Here's the drawing with two shaded views (mm, measured from the low corner). I have some questions. Coordinates: 2 decimals unless noted, no trailing zeros. Write each loop counter-clockwise with the first axis right and the second up, starting at its lowest first coordinate (ties: lowest second). Pieces come first, ordered by that corner, then holes. Notation, with made-up numbers: (-31.75, 76) -> (2.25, 76) arc R33 cw to (2.25, 112) -> close; hole circle Ø7 at (68.25, 30). An arc over 180 degrees is marked (long way). Use one line per item in the form item = value.
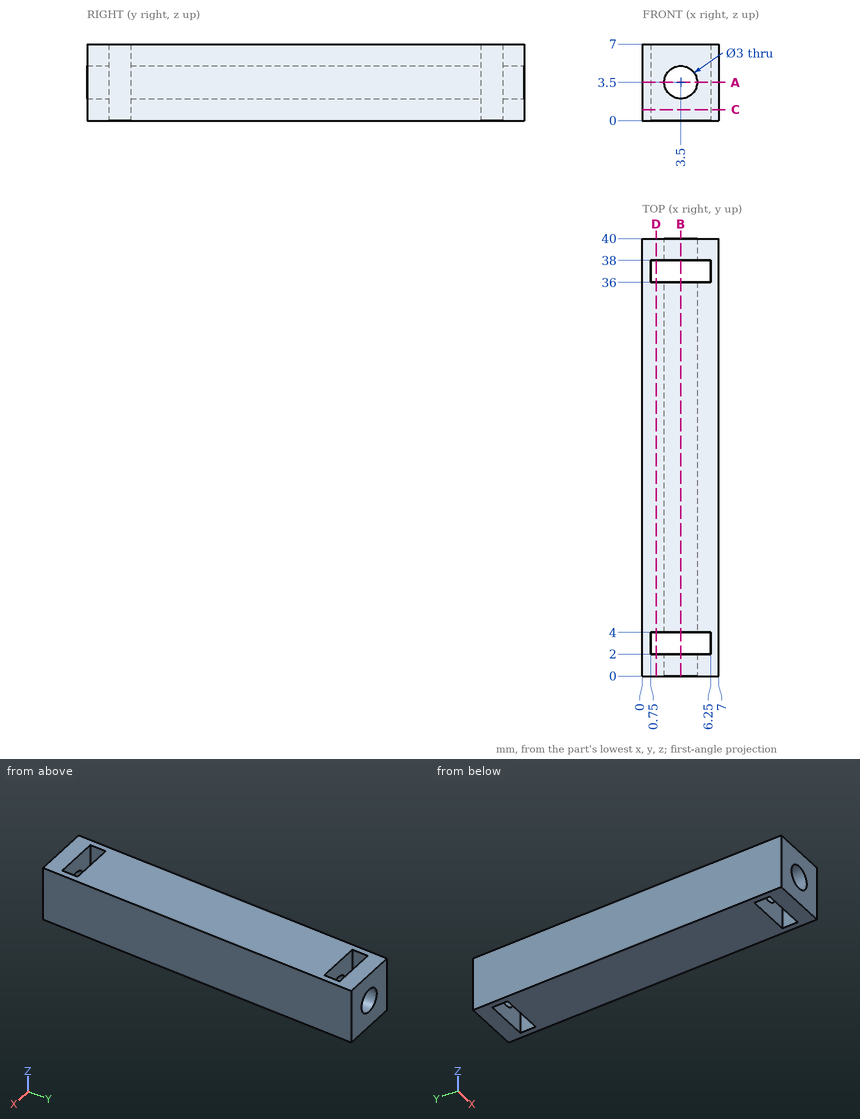
Q1. Suppose I cut it at B-B (x = 3.5). Write out the boundary of the cut face in (y, z), then the cut area to 3 significant figures.
Return value:
outline = (0, 0) -> (2, 0) -> (2, 2) -> (0, 2) -> close; (0, 5) -> (2, 5) -> (2, 7) -> (0, 7) -> close; (4, 0) -> (36, 0) -> (36, 2) -> (4, 2) -> close; (4, 5) -> (36, 5) -> (36, 7) -> (4, 7) -> close; (38, 0) -> (40, 0) -> (40, 2) -> (38, 2) -> close; (38, 5) -> (40, 5) -> (40, 7) -> (38, 7) -> close
area = 144 mm2
Q2. Suppose I cut it at D-D (x = 1.25). Write out the boundary of the cut face in (y, z), then the cut area to 3 significant figures.
Return value:
outline = (0, 0) -> (2, 0) -> (2, 7) -> (0, 7) -> close; (4, 0) -> (36, 0) -> (36, 7) -> (4, 7) -> close; (38, 0) -> (40, 0) -> (40, 7) -> (38, 7) -> close
area = 252 mm2
Q3. Suppose I cut it at A-A (z = 3.5). Write out the boundary of the cut face in (x, y).
Return value:
outline = (0, 0) -> (2, 0) -> (2, 2) -> (0.75, 2) -> (0.75, 4) -> (2, 4) -> (2, 36) -> (0.75, 36) -> (0.75, 38) -> (2, 38) -> (2, 40) -> (0, 40) -> close; (5, 0) -> (7, 0) -> (7, 40) -> (5, 40) -> (5, 38) -> (6.25, 38) -> (6.25, 36) -> (5, 36) -> (5, 4) -> (6.25, 4) -> (6.25, 2) -> (5, 2) -> close
Q4. Suppose I cut it at C-C (z = 1). Write out the boundary of the cut face in (x, y).
Return value:
outline = (0, 0) -> (7, 0) -> (7, 40) -> (0, 40) -> close; hole (0.75, 2) -> (6.25, 2) -> (6.25, 4) -> (0.75, 4) -> close; hole (0.75, 36) -> (6.25, 36) -> (6.25, 38) -> (0.75, 38) -> close
Q5. If I drill on line 1 (Y direction, x = 4.5, z = 1); line 2 (X direction, y = 14.5, z = 3.5), over which ranges is the centre line in solid material (lowest first)? Write a range as from..to.
Return value:
line_1 = 0..2, 4..36, 38..40
line_2 = 0..2, 5..7
